Part model, mm, in its own coordinate system. A direction names the side the tool comes from. Coordinates: 2 decimals unless noted, no trailing zeros. Write item = value, one per line. Start each with the question number.
Q1. Band-saw the part on A-A, the plane z = 2.2. Give the number of separate pieces and of enclosed holes in the cut face, plus the area to 3 significant figures.
Q2. Pin check, flat tips, straight feed: P1, Ø1.2, axis at x = 39.5, z = 1, coming from the +Y side; P2, Ø1, axis at x = 15, z = 1.5, coming from the -Y side; P3, Ø1, axis at y = -18.5, z = 2, coming from the +X side. Stop position of each tip, or through.
Q3. Probe line 1 (X direction, y = 10.5, z = 2.65); line 2 (Y direction, x = -97.4, z = 1.7). List the from-to ranges inside material, lowest first.
Q4. Tool access for faces 1 (the flat face through (-87.5, 19, 2)), 2 (the flat face through (-95, -17.64, 2)), 3 (the flat face through (87.5, -19, 2)), 4 (the flat face through (51, 17.64, 2)), 5 (the flat face through (51, -17.64, 2)): list every direction of +Z, -Z, +X, -X, +Y, -Y with a clear straight run to the whole face (end or side of a thin tool).
Q5. Pull direction X, two halves, no side cores. Call faces 6 (the flat face through (35.95, 16, 2)), 7 (the flat face through (-51, 17.64, 2)), 8 (the flat face through (87.5, 19, 2)), 9 (the flat face through (-87.5, -19, 2)): released by +X, released by -X, zero draft, split by the parting line, or undercut.
from build123d import *

# Parameters (mm, degrees)
F1_W     = 206
F1_H     = 35.28
F2_DEPTH = 3.2
F3_W     = 25
F3_H     = 3.2
F4_DEPTH = 3.2
F5_R     = 1.55
F5_W     = 3.1
F5_H     = 3.75
F5_H_2   = 2.5
F5_W_2   = 1.1
F5_H_3   = 2.75
F6_DEPTH = 3.201


with BuildPart() as f2:
    # F1 (on Top) → F2 (new body)
    with BuildSketch(Plane.XY):
        Rectangle(F1_W, F1_H)
    extrude(amount=F2_DEPTH)

    # F3 (on face) → F4 (join, through all)
    with BuildSketch(Plane.XY.offset(3.2)):
        with Locations((-75, -19.24)):
            Rectangle(F3_W, F3_H)
        with Locations((0, -19.24)):
            Rectangle(F3_W, F3_H)
        with Locations((75, -19.24)):
            Rectangle(F3_W, F3_H)
        with Locations((75, 19.24)):
            Rectangle(F3_W, F3_H)
        with Locations((-75, 19.24)):
            Rectangle(F3_W, F3_H)
        with Locations((0, 19.24)):
            Rectangle(F3_W, F3_H)
    extrude(amount=-F4_DEPTH)

    # F5 (on face) → F6 (cut, through all)
    with BuildSketch(Plane.XY.offset(3.2)):
        with Locations((-97.4, 0)):
            Circle(F5_R)
        with Locations((97.4, 0)):
            Circle(F5_R)
        with Locations((-37.5, -15.765)):
            Rectangle(F5_W, F5_H)
        with Locations((-37.5, -12.64)):
            Rectangle(F5_W, F5_H_2)
        with Locations((-35.4, -12.64)):
            Rectangle(F5_W_2, F5_H_2)
        with Locations((-37.5, -10.015)):
            Rectangle(F5_W, F5_H_3)
        with Locations((-39.6, -12.64)):
            Rectangle(F5_W_2, F5_H_2)
        with Locations((37.5, -15.765)):
            Rectangle(F5_W, F5_H)
        with Locations((37.5, -12.64)):
            Rectangle(F5_W, F5_H_2)
        with Locations((35.4, -12.64)):
            Rectangle(F5_W_2, F5_H_2)
        with Locations((39.6, -12.64)):
            Rectangle(F5_W_2, F5_H_2)
        with Locations((37.5, -10.015)):
            Rectangle(F5_W, F5_H_3)
        with Locations((-37.5, 10.015)):
            Rectangle(F5_W, F5_H_3)
        with Locations((-35.4, 12.64)):
            Rectangle(F5_W_2, F5_H_2)
        with Locations((-37.5, 12.64)):
            Rectangle(F5_W, F5_H_2)
        with Locations((-39.6, 12.64)):
            Rectangle(F5_W_2, F5_H_2)
        with Locations((-37.5, 15.765)):
            Rectangle(F5_W, F5_H)
        with Locations((39.6, 12.64)):
            Rectangle(F5_W_2, F5_H_2)
        with Locations((37.5, 10.015)):
            Rectangle(F5_W, F5_H_3)
        with Locations((37.5, 12.64)):
            Rectangle(F5_W, F5_H_2)
        with Locations((37.5, 15.765)):
            Rectangle(F5_W, F5_H)
        with Locations((35.4, 12.64)):
            Rectangle(F5_W_2, F5_H_2)
    extrude(amount=-F6_DEPTH, mode=Mode.SUBTRACT)


solid = f2.part
Ans:
q1.separate_pieces = 1
q1.enclosed_holes = 2
q1.area = 7,600 mm2
q2.P1 = 17.64
q2.P2 = -17.64
q2.P3 = 87.5
q3.line_1 = -103 to -39.05, -35.95 to 35.95, 39.05 to 103
q3.line_2 = -17.64 to -1.55, 1.55 to 17.64
q4.face_1 = +Z, -Z, -X, +Y
q4.face_2 = +Z, -Z, -X, -Y
q4.face_3 = +Z, -Z, +X, -Y
q4.face_4 = +Z, -Z, +Y
q4.face_5 = +Z, -Z, -Y
q5.face_6 = undercut
q5.face_7 = undercut
q5.face_8 = released by +X
q5.face_9 = released by -X
